```python
from build123d import *

# Parameters (mm, degrees)
BOSS_EXTRUDE1_DEPTH      = 8
BOSS_EXTRUDE1_DEPTH_BACK = 8


with BuildPart() as part:
    # Sketch1 → Boss-Extrude1 (new, two sides: drawn at the far end of the back side and taken through both)
    with BuildSketch(Plane.XY.offset(-BOSS_EXTRUDE1_DEPTH_BACK)):
        with BuildLine():
            Line((-23.041785381, -271.526308081), (-23.041785381, -283))
            ThreePointArc((-23.041785381, -283), (-22.163105725, -285.121320344), (-20.041785381, -286))
            Line((-20.041785381, -286), (-11.041785381, -286))
            ThreePointArc((-11.041785381, -286), (-8.213358256, -284.828427125), (-7.041785381, -282))
            Line((-7.041785381, -282), (-7.041785381, -255.150929215))
            ThreePointArc((-7.041785381, -255.150929215), (-7.920465038, -253.029608872), (-10.041785381, -252.150929215))
            Line((-10.041785381, -252.150929215), (-20.041785381, -252.150929215))
            ThreePointArc((-20.041785381, -252.150929215), (-22.163105725, -253.029608872), (-23.041785381, -255.150929215))
            Line((-23.041785381, -255.150929215), (-23.041785381, -257.783091126))
            Line((-23.041785381, -257.783091126), (-22.041785381, -257.783091126))
            Line((-22.041785381, -257.783091126), (-22.041785381, -255.150929215))
            ThreePointArc((-22.041785381, -255.150929215), (-21.455998944, -253.736715653), (-20.041785381, -253.150929215))
            Line((-20.041785381, -253.150929215), (-10.041785381, -253.150929215))
            ThreePointArc((-10.041785381, -253.150929215), (-8.627571819, -253.736715653), (-8.041785381, -255.150929215))
            Line((-8.041785381, -255.150929215), (-8.041785381, -282))
            ThreePointArc((-8.041785381, -282), (-8.920465038, -284.121320344), (-11.041785381, -285))
            Line((-11.041785381, -285), (-20.041785381, -285))
            ThreePointArc((-20.041785381, -285), (-21.455998944, -284.414213562), (-22.041785381, -283))
            Line((-22.041785381, -283), (-22.041785381, -271.526308081))
            Line((-22.041785381, -271.526308081), (-23.041785381, -271.526308081))
        make_face()
    extrude(amount=BOSS_EXTRUDE1_DEPTH + BOSS_EXTRUDE1_DEPTH_BACK)


solid = part.part
```
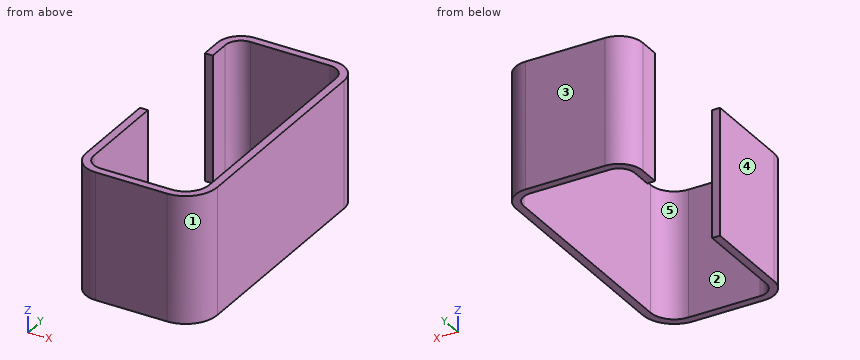
Build history of the part. All positions in model axes, mm. Face numbers are marked on the shaded views. A direction names the side the tool comes from. Coordinates: 2 decimals unless noted, no trailing zeros. Order: outer loops, then holes, each group sorted by start corner. A loop starts at its lowest first (then second) coordinate and runs counter-clockwise, first axis right, second up. Notation, with made-up numbers: M 19,75 L 55,75 A29 ccw 55,105 Z; hole C -11,-8 d2. An arc over 180 degrees is marked long. One line per question, with ' | ' between items. Start each with the question number.
1. Cut at A-A (y = -277). Write the cut outline in (x, z).
2. Cut at B-B (x = -18). Write the cut outline in (y, z).
3. Tool access for the marked faces 1 and 2: list every direction of +Z, -Z, +X, -X, +Y, -Y with a clear straight run to the whole face (end or side of a thin tool).
4. Cut at D-D (y = -264). Write the cut outline in (x, z).
5. Wall check: line 1 along X through (y, z) = (-256, -1.75); line 2 along Y through (x, z) = (-12, -1.5); line 3 along X through (y, z) = (-260, -5.75). Give the ranges that are in metal, low to high. Write a range as [from, to].
6. Cut at C-C (z = -1.25). Write the cut outline in (x, y), plus the area to 3 significant figures.
7. Mould opens along X. For the marked faces 3, 4 and 5 say: +X half, -X half, draft (parallel to the pull), parting line (faces both ways), or undercut.
8. Flat gauge pin, fed straight in: P1, Ø0.5, axis at x = -22.5, z = -3, coming from the +Y side. Where does the tip first touch, or does it go through?
The answers:
1) outline: M -23.04,-8 L -22.04,-8 L -22.04,8 L -23.04,8 Z; M -8.04,-8 L -7.04,-8 L -7.04,8 L -8.04,8 Z
2) outline: M -286,-8 L -285,-8 L -285,8 L -286,8 Z; M -253.15,-8 L -252.15,-8 L -252.15,8 L -253.15,8 Z
3) face 1: +Z, -Z, +X, -Y | face 2: +Z, -Z
4) outline: M -8.04,-8 L -7.04,-8 L -7.04,8 L -8.04,8 Z
5) line 1: x = [-23.04, -22.04], [-8.04, -7.04] | line 2: y = [-286, -285], [-253.15, -252.15] | line 3: x = [-8.04, -7.04]
6) outline: M -23.04,-283 A3 ccw -20.04,-286 L -11.04,-286 A4 ccw -7.04,-282 L -7.04,-255.15 A3 ccw -10.04,-252.15 L -20.04,-252.15 A3 ccw -23.04,-255.15 L -23.04,-257.78 L -22.04,-257.78 L -22.04,-255.15 A2 cw -20.04,-253.15 L -10.04,-253.15 A2 cw -8.04,-255.15 L -8.04,-282 A3 cw -11.04,-285 L -20.04,-285 A2 cw -22.04,-283 L -22.04,-271.53 L -23.04,-271.53 Z | area: 77.2 mm2
7) face 3: draft | face 4: -X half | face 5: undercut
8) P1: stops at y = -253.12
